from build123d import *


with BuildPart() as f1:
    # F0 (on Right) → F1 (revolve)
    with BuildSketch(Plane.YZ):
        with BuildLine():
            Line((0, 5.89504), (0, 13.952179))
            Line((0, 13.952179), (-3, 13.952179))
            ThreePointArc((-3, 13.952179), (-3.707107, 13.659285), (-4, 12.952179))
            Line((-4, 12.952179), (-4, 11.952179))
            Line((-4, 11.952179), (-2, 11.952179))
            Line((-2, 11.952179), (-2, 7.952179))
            Line((-2, 7.952179), (-2.96099, 7.952179))
            Line((-2.96099, 7.952179), (-3.330959, 7.452179))
            Line((-3.330959, 7.452179), (-2, 7.452179))
            Line((-2, 7.452179), (-2, 0.852179))
            ThreePointArc((-2, 0.852179), (-1.853553, 0.498625), (-1.5, 0.352179))
            Line((-1.5, 0.352179), (-0.825782, 0.352179))
            Line((-0.825782, 0.352179), (-0.825782, 5.89504))
            Line((-0.825782, 5.89504), (0, 5.89504))
        make_face()
    revolve(axis=Axis((0, 0, 9.923609), (0, 0, -1)))


solid = f1.part
CAD build for the part. Positions are in the model's coordinates, mm. A direction names the side the tool comes from. Give positions to 0.01 mm unless a question says otherwise; leave off trailing zeros. Write each loop counter-clockwise with the first axis right and the second up, starting at its lowest first coordinate (ties: lowest second). Pieces come first, ordered by that corner, then holes. Notation, with made-up numbers: (66, 38.5) - (92, 38.5) arc R15 cw to (92, 50.5) - close; hole circle Ø7 at (-11, -26). An arc over 180 degrees is marked (long way). Put each result on its own line as item: value.
(1) Saw through at C-C (z = 4.75). List the corners of the cut face in (x, y), then the cut area to 3 significant figures.
Working result:
outline: circle Ø4 at (0, 0); hole circle Ø1.65 at (0, 0)
area: 10.4 mm^2
(2) Pull direction Z, two halves, no side cores. Call faces 1 (the flat face through (1, 2, 11.952)), 2 (the flat face through (2.2, 0, 7.452)), 3 (the cylindrical face through (2, 0, 10)), 4 (the cylindrical face through (3.905, 0.867, 12.445)): released by +Z, released by -Z, zero draft, split by the parting line, or undercut.
Working result:
face 1: undercut
face 2: released by -Z
face 3: undercut
face 4: zero draft
(3) Tool access for faces 5 (the flat face through (1, 0, 0.352)), 6 (the cylindrical face through (0.8, 0.2, 3.2)), 7 (the flat face through (2, 1, 7.952)): list every direction of +Z, -Z, +X, -X, +Y, -Y with a clear straight run to the whole face (end or side of a thin tool).
Working result:
face 5: -Z, +X, -X, +Y, -Y
face 6: -Z
face 7: none
(4) Saw through at D-D (z = 8.75). List the corners of the cut face in (x, y), then the cut area to 3 significant figures.
Working result:
outline: circle Ø4 at (0, 0)
area: 12.6 mm^2
(5) Saw through at A-A (x = 0). List the corners of the cut face in (y, z), then the cut area to 3 significant figures.
Working result:
outline: (-4, 11.95) - (-2, 11.95) - (-2, 7.95) - (-2.96, 7.95) - (-3.33, 7.45) - (-2, 7.45) - (-2, 0.85) arc R0.5 ccw to (-1.5, 0.35) - (-0.83, 0.35) - (-0.83, 5.9) - (0.83, 5.9) - (0.83, 0.35) - (1.5, 0.35) arc R0.5 ccw to (2, 0.85) - (2, 7.45) - (3.33, 7.45) - (2.96, 7.95) - (2, 7.95) - (2, 11.95) - (4, 11.95) - (4, 12.95) arc R1 ccw to (3, 13.95) - (-3, 13.95) arc R1 ccw to (-4, 12.95) - close
area: 53.9 mm^2
(6) Wall check: L1, parallel to Z at x = 2.25, y = -0.75; L2, parallel to X at y = 0, z = 3.65. Give the ranges that are in metal, low to high.
Working result:
L1: 7.45 to 7.95, 11.95 to 13.95
L2: -2 to -0.83, 0.83 to 2
(7) Drop flat-ended pins along their axis: pin 1 Ø4 at (x, z) = (3, 2) entering from -Y; pin 2 Ø1.5 at (x, z) = (1.5, 9) entering from +Y; pin 3 Ø1.5 at (y, z) = (0, 10) entering from -X. Give the stop position or say it passes through.
Working result:
pin 1: y = -1.73
pin 2: y = 1.85
pin 3: x = -2
